The model under review builds one solid part; all positions refer to its coordinate system, in mm. A direction names the side the tool comes from. Give positions to 0.01 mm unless a question says otherwise; leave off trailing zeros. Put each result on its own line as item: value. Start each with the question number.
from build123d import *

# Parameters (mm, degrees)
CUT_EXTRUDE1_START = 2.2987
CUT_EXTRUDE1_DEPTH = 10.922
CIRPATTERN1_COUNT  = 10
CHAMFER1_SIZE      = 0.5


with BuildPart() as part:
    # Sketch2 → Revolve1 (revolve)
    with BuildSketch(Plane(origin=(0, 0, 0), x_dir=(0, 0, -1), z_dir=(1, 0, 0)), mode=Mode.PRIVATE) as revolve1_sk:
        with BuildLine():
            Line((-3.9878, 3.175), (10.3124, 3.175))
            Line((10.3124, 3.175), (10.3124, 11.1125))
            Line((10.3124, 11.1125), (9.46785, 11.1125))
            ThreePointArc((9.46785, 11.1125), (8.846862309, 10.395787163), (8.6233, 9.4742))
            Line((8.6233, 9.4742), (8.6233, 7.8359))
            Line((8.6233, 7.8359), (-2.2987, 7.8359))
            Line((-2.2987, 7.8359), (-2.2987, 9.4742))
            ThreePointArc((-2.2987, 9.4742), (-2.522262309, 10.395787163), (-3.14325, 11.1125))
            Line((-3.14325, 11.1125), (-3.9878, 11.1125))
            Line((-3.9878, 11.1125), (-3.9878, 3.175))
        make_face()
    revolve(revolve1_sk.sketch.rotate(Axis((0, 0, 10.3124), (0, 0, -1)), 90), axis=Axis((0, 0, 10.3124), (0, 0, -1)))

    # Sketch3 → Cut-Extrude1 (cut)
    with BuildSketch(Plane.XY.offset(CUT_EXTRUDE1_START)):
        with BuildLine():
            Line((-0.635, 6.329348022), (0.635, 6.329348022))
            Line((0.635, 6.329348022), (1.287830721, 7.729348022))
            ThreePointArc((1.287830721, 7.729348022), (0, 7.8359), (-1.287830721, 7.729348022))
            Line((-1.287830721, 7.729348022), (-0.635, 6.329348022))
        make_face()
    cut_extrude1 = extrude(amount=-CUT_EXTRUDE1_DEPTH, mode=Mode.SUBTRACT)

    # CirPattern1: Cut-Extrude1 ×10 about axis
    cirpattern1_axis = Axis((0, 0, 0), (0, 0, 1))
    for i in range(1, CIRPATTERN1_COUNT):
        add(cut_extrude1.rotate(cirpattern1_axis, i * 360 / CIRPATTERN1_COUNT), mode=Mode.SUBTRACT)

    # Chamfer1
    chamfer1_edges = [part.edges().sort_by_distance(p)[0] for p in [
        (-11.1125, 0, -10.3124),
        (-3.175, 0, -10.3124),
        (-3.175, 0, 3.9878),
        (-11.1125, 0, 3.9878),
    ]]
    chamfer(chamfer1_edges, length=CHAMFER1_SIZE)


solid = part.part
(1) Insertion check: pin 1 (0.6 mm diameter, centred on x = 0.5, z = -5.5, fed in from -Y); pin 2 (1 mm diameter, centred on x = 2, z = -0.5, fed in from -Y); pin 3 (2 mm diameter, centred on x = 1.5, z = -4.5, fed in from +Y). Each pin has a flat end and moves straight along its axis. Give the tip position at first contact, or say it passes through.
(2) To check wall thickness, follow L1, parallel to Z at x = -6, y = 6; L2, parallel to Y at x = 0, z = -3 (3 decimals); L3, parallel to X at y = 5, z = -6.25. State the ranges of each line that lie inside material, in increasing order. Write a range as [from, to].
(3) For faces 1 (the flat face through (-4.9, -5.117, -3.086)), 2 (the cylindrical face through (7.836, 0.016, -3.086)), 3 (the flat face through (-3.727, 5.115, -3.086)), 4 (the cylindrical face through (-7.836, -0.016, -3.086)), list the 3-axis set-ups (+Z, -Z, +X, -X, +Y, -Y) from which the entire face can be reached by the end or side of a thin tool; tool diameter is ignored.
(4) Draft analysis for pull direction X (two halves, no side actions). For faces 5 (the flat face through (-3.71, -5.13, -3.09)), 6 (the flat face through (3.35, -6.24, -3.09)), 7 (the flat face through (5, 0, 3.988)), 8 (the flat face through (-6.02, -1.96, -3.09)), state which applies: +X half, -X half, draft (parallel to the pull), parting line (faces both ways), or undercut.
Check sheet entries:
1. pin 1: stops at y = -6.68
1. pin 2: stops at y = -7.69
1. pin 3: stops at y = 7.73
2. L1: z = [-10.31, -8.62], [2.3, 3.99]
2. L2: y = [-6.329, -3.175], [3.175, 6.329]
2. L3: x = [-6.03, -4.69], [-3.89, 3.89], [4.69, 6.03]
3. face 1: -Y
3. face 2: +X
3. face 3: none
3. face 4: -X
4. face 5: undercut
4. face 6: +X half
4. face 7: draft
4. face 8: -X half
